```python
from build123d import *

# Parameters (mm, degrees)
BOSS_EXTRUDE1_DEPTH = 63.5
SKETCH2_R           = 13
SKETCH2_R_2         = 2
CUT_EXTRUDE1_DEPTH  = 5
SKETCH3_R           = 2.5
CUT_EXTRUDE2_DEPTH  = 5


with BuildPart() as part:
    # Sketch1 → Boss-Extrude1 (new body)
    with BuildSketch(Plane.XY):
        with BuildLine():
            Line((0, 0), (0, 60))
            Line((0, 60), (80, 60))
            Line((80, 60), (80, 55))
            Line((80, 55), (10, 55))
            ThreePointArc((10, 55), (6.464466094, 53.535533906), (5, 50))
            Line((5, 50), (5, 0))
            Line((5, 0), (0, 0))
        make_face()
    extrude(amount=BOSS_EXTRUDE1_DEPTH)

    # Sketch2 → Cut-Extrude1 (cut)
    with BuildSketch(Plane.ZY):
        with Locations((31.75, 30)):
            Circle(SKETCH2_R)
        with Locations((49.5, 30)):
            Circle(SKETCH2_R_2)
        with Locations((31.75, 12.25)):
            Circle(SKETCH2_R_2)
        with Locations((14, 30)):
            Circle(SKETCH2_R_2)
        with Locations((31.75, 47.75)):
            Circle(SKETCH2_R_2)
    extrude(amount=-CUT_EXTRUDE1_DEPTH, mode=Mode.SUBTRACT)

    # Sketch3 → Cut-Extrude2 (cut)
    with BuildSketch(Plane(origin=(0, 60, 0), x_dir=(1, 0, 0), z_dir=(0, 1, 0))):
        with Locations((15, -15.875)):
            Circle(SKETCH3_R)
        with Locations((65, -15.875)):
            Circle(SKETCH3_R)
        with Locations((65, -47.625)):
            Circle(SKETCH3_R)
        with Locations((15, -47.625)):
            Circle(SKETCH3_R)
    extrude(amount=-CUT_EXTRUDE2_DEPTH, mode=Mode.SUBTRACT)


solid = part.part
```
Check sheet for the modelled part. Datum: model origin and axes. Units: mm. A direction names the side the tool comes from. Give positions to 0.01 mm unless a question says otherwise; leave off trailing zeros. Write each loop counter-clockwise with the first axis right and the second up, starting at its lowest first coordinate (ties: lowest second). Pieces come first, ordered by that corner, then holes.
Item 1: Access from +Z, -Z, +X, -X, +Y, -Y to the whole of each face (thin tool, end or side, straight path). Record for faces 5 (the face through (13.02, 57.54, 17.4)), 6 (the face through (5, 14, 24)).
Item 2: Scan lines: L1, parallel to Z at x = 15, y = 58.1 (3 decimals); L2, parallel to Y at x = 1.15, z = 31.75; L3, parallel to Y at x = 53, z = 35.5. Record each from-to range of solid material in increasing order.
Item 3: Draft check along Y on faces 1 (the face through (2.465, 30.572, 18.763)), 2 (the face through (2.465, 12.851, 33.658)), 3 (the face through (67.385, 57.535, 15.124)), 4 (the face through (45, 55, 31)). Enter one of: released by +Y, released by -Y, zero draft, split by the parting line, or undercut.
Item 4: Cross-section at D-D (y = 30). Enter the section's corners in (x, z).
Item 5: Gauge pin test, flat ends, axial feed: pin 1 (5 mm diameter, centred on x = 9.5, z = 20, fed in from -Y); pin 2 (5 mm diameter, centred on x = 70.5, z = 16.5, fed in from -Y); pin 3 (3 mm diameter, centred on y = 47.75, z = 31.75, fed in from +X); pin 4 (4.5 mm diameter, centred on y = 30, z = 14, fed in from -X). Record the tip position at first contact, or that the pin passes through.
Item 6: Cross-section at A-A (z = 31.75). Enter the section's corners in (x, y), and give its area (3 significant figures).
Item 7: Cross-section at C-C (y = 39.5). Enter the section's corners in (x, z).
Item 8: Cross-section at B-B (x = 15). Enter the section's corners in (y, z) (3 decimals), and give its area (4 significant figures).
Report:
1. face 5: +Y, -Y
1. face 6: +Z, -Z, +X, -Y
2. L1: z = 0 to 13.375, 18.375 to 45.125, 50.125 to 63.5
2. L2: y = 0 to 10.25, 14.25 to 17, 43 to 45.75, 49.75 to 60
2. L3: y = 55 to 60
3. face 1: undercut
3. face 2: undercut
3. face 3: zero draft
3. face 4: released by -Y
4. outline: (0, 0) - (5, 0) - (5, 12) - (0, 12) - close; (0, 16) - (5, 16) - (5, 18.75) - (0, 18.75) - close; (0, 44.75) - (5, 44.75) - (5, 47.5) - (0, 47.5) - close; (0, 51.5) - (5, 51.5) - (5, 63.5) - (0, 63.5) - close
5. pin 1: stops at y = 54
5. pin 2: stops at y = 55
5. pin 3: passes through
5. pin 4: stops at x = 0
6. outline: (0, 0) - (5, 0) - (5, 10.25) - (0, 10.25) - close; (0, 14.25) - (5, 14.25) - (5, 17) - (0, 17) - close; (0, 43) - (5, 43) - (5, 45.75) - (0, 45.75) - close; (0, 49.75) - (5, 49.75) - (5, 50) arc R5 cw to (10, 55) - (80, 55) - (80, 60) - (0, 60) - close
6. area: 510 mm2
7. outline: (0, 0) - (5, 0) - (5, 22.88) - (0, 22.88) - close; (0, 40.62) - (5, 40.62) - (5, 63.5) - (0, 63.5) - close
8. outline: (55, 0) - (60, 0) - (60, 13.375) - (55, 13.375) - close; (55, 18.375) - (60, 18.375) - (60, 45.125) - (55, 45.125) - close; (55, 50.125) - (60, 50.125) - (60, 63.5) - (55, 63.5) - close
8. area: 267.5 mm2
